Geometry check sheet. Reference: the model listing, model coordinates, mm. A direction names the side the tool comes from. Give positions to 0.01 mm unless a question says otherwise; leave off trailing zeros. Write each loop counter-clockwise with the first axis right and the second up, starting at its lowest first coordinate (ties: lowest second). Pieces come first, ordered by that corner, then holes. Notation, with made-up numbers: (-4.5, -15.5) -> (15.5, -15.5) arc R15 cw to (15.5, -5.5) -> close; hole circle Ø8 at (59.25, -34.75). An arc over 180 degrees is marked (long way). Write item = value, one per line. Start each with the question number.
1. Cross-section at C-C, the plane z = 2.75. Record the cut outline in (x, y).
2. Mould release check, pull along Z, two halves, no side actions. Record for faces 6 (the flat face through (25, -3, 7)), 7 (the flat face through (7, -14, 14)), 8 (the flat face through (21, -6, 7)): pulls with the +Z half, pulls with the -Z half, needs draft (parallel to the pull), parting line crosses it, or undercut.
3. Depth check by flat-ended pin: P1, Ø2, axis at x = 18.5, z = 9.5, coming from the -Y side; P2, Ø2, axis at y = -17.5, z = 6, coming from the +X side; P3, Ø5.5, axis at y = -17.78, z = 7, coming from the -X side; P4, Ø6, axis at x = 13.5, y = -32.5, coming from the +Z side. Enter the tip coordinate at first touch or a pass-through.
4. Cross-section at A-A, the plane z = 7. Record the cut outline in (x, y), plus the area to 3 significant figures.
5. Cross-section at B-B, the plane y = -1. Record the cut outline in (x, z).
6. Thickness scan on line 1 along Y through (x, z) = (2.4, 7); line 2 along Z through (x, y) = (19.5, -16.5); line 3 along X through (y, z) = (-38, 4.25). Record the ranges inside material, lowest first.
7. Set-up check for faces 1 (the flat face through (-9.5, 5, 7)), 2 (the cylindrical face through (8.281, -8.406, 7.074)), 3 (the flat face through (-2, 3, 7)), 4 (the flat face through (16.405, -23.681, 0.838)), 5 (the flat face through (0, -25, 7)): record each of +Z, -Z, +X, -X, +Y, -Y from which the full face is reachable in a straight line by a thin tool's end or side.
8. Cross-section at D-D, the plane x = -11.5. Record the cut outline in (y, z).
```python
from build123d import *

# Parameters (mm, degrees)
BOSS_EXTRUDE1_DEPTH = 14
SKETCH2_R           = 1.7
CUT_EXTRUDE1_DEPTH  = 10
SKETCH3_R           = 1.7
CUT_EXTRUDE2_DEPTH  = 10
SKETCH14_W          = 14
SKETCH14_H          = 6
BOSS_EXTRUDE3_DEPTH = 14
FILLET8_R           = 2
SKETCH17_W          = 1.5
SKETCH17_H          = 1.7
SKETCH18_W          = 19
SKETCH18_H          = 1.7
SKETCH20_W          = 19
SKETCH20_H          = 1.7
SKETCH19_W          = 1.5
SKETCH19_H          = 1.7
FILLET9_R           = 8
SKETCH21_W          = 7.5
SKETCH21_H          = 7
BOSS_EXTRUDE4_DEPTH = 14
FILLET10_R          = 4
FILLET11_R          = 2
FILLET12_R          = 2


with BuildPart() as part:
    # Sketch1 → Boss-Extrude1 (new body)
    with BuildSketch(Plane.XY):
        Polygon((0, 0), (25, 0), (25, -6), (6, -6), (6, -42), (0, -42), (0, -5.547169811), align=None)
    extrude(amount=BOSS_EXTRUDE1_DEPTH)

    # Sketch2 → Cut-Extrude1 (cut)
    with BuildSketch(Plane(origin=(6, 0, 0), x_dir=(0, 0, -1), z_dir=(1, 0, 0))):
        with Locations((-7, -17.78)):
            Circle(SKETCH2_R)
        with Locations((-7, -34.058)):
            Circle(SKETCH2_R)
    extrude(amount=-CUT_EXTRUDE1_DEPTH, mode=Mode.SUBTRACT)

    # Sketch3 → Cut-Extrude2 (cut)
    with BuildSketch(Plane.XZ.offset(6)):
        with Locations((18.3, 7)):
            Circle(SKETCH3_R)
    extrude(amount=-CUT_EXTRUDE2_DEPTH, mode=Mode.SUBTRACT)

    # Sketch14 → Boss-Extrude3 (add)
    with BuildSketch(Plane(origin=(0, 0, 0), x_dir=(-1, 0, 0), z_dir=(0, 0, -1))):
        with Locations((7, -3)):
            Rectangle(SKETCH14_W, SKETCH14_H)
    extrude(amount=-BOSS_EXTRUDE3_DEPTH)

    # Fillet8
    fillet8_edges = [part.edges().sort_by_distance(p)[0] for p in [
        (0, -6, 7),
    ]]
    fillet(fillet8_edges, radius=FILLET8_R)

    # Sketch17 → Loft2 section 0
    with BuildSketch(Plane.XZ.offset(42)):
        with Locations((6.75, 13.15)):
            Rectangle(SKETCH17_W, SKETCH17_H)
    # Sketch18 → Loft2 section 1
    with BuildSketch(Plane.XZ.offset(6)):
        with Locations((15.5, 13.15)):
            Rectangle(SKETCH18_W, SKETCH18_H)
    loft()

    # Sketch20 → Loft3 section 0
    with BuildSketch(Plane.XZ.offset(6)):
        with Locations((15.5, 0.85)):
            Rectangle(SKETCH20_W, SKETCH20_H)
    # Sketch19 → Loft3 section 1
    with BuildSketch(Plane.XZ.offset(42)):
        with Locations((6.75, 0.85)):
            Rectangle(SKETCH19_W, SKETCH19_H)
    loft()

    # Fillet9
    fillet9_edges = [part.edges().sort_by_distance(p)[0] for p in [
        (6, -6, 7),
    ]]
    fillet(fillet9_edges, radius=FILLET9_R)

    # Sketch21 → Boss-Extrude4 (add)
    with BuildSketch(Plane(origin=(0, 0, 0), x_dir=(-1, 0, 0), z_dir=(0, 0, -1))):
        with Locations((5.75, 3.5)):
            Rectangle(SKETCH21_W, SKETCH21_H)
    extrude(amount=-BOSS_EXTRUDE4_DEPTH)

    # Fillet10
    fillet10_edges = [part.edges().sort_by_distance(p)[0] for p in [
        (-9.5, 0, 7),
    ]]
    fillet(fillet10_edges, radius=FILLET10_R)

    # Fillet11
    fillet11_edges = [part.edges().sort_by_distance(p)[0] for p in [
        (7.5, -42, 0.85),
    ]]
    fillet(fillet11_edges, radius=FILLET11_R)

    # Fillet12
    fillet12_edges = [part.edges().sort_by_distance(p)[0] for p in [
        (7.5, -42, 13.15),
    ]]
    fillet(fillet12_edges, radius=FILLET12_R)


solid = part.part
```
Answers:
q1.outline = (-14, -6) -> (-2, -6) arc R2 cw to (0, -8) -> (0, -42) -> (6, -42) -> (6, -14) arc R8 cw to (14, -6) -> (25, -6) -> (25, 0) -> (-2, 0) -> (-2, 7) -> (-9.5, 7) -> (-9.5, 4) arc R4 cw to (-13.5, 0) -> (-14, 0) -> close
q2.face_6 = needs draft
q2.face_7 = pulls with the +Z half
q2.face_8 = undercut
q3.P1 = -6
q3.P2 = 6
q3.P3 = 0
q3.P4 = 14
q4.outline = (-14, -6) -> (-2, -6) arc R2 cw to (0, -8) -> (0, -16.08) -> (6, -16.08) -> (6, -14) arc R8 cw to (14, -6) -> (16.6, -6) -> (16.6, 0) -> (-2, 0) -> (-2, 7) -> (-9.5, 7) -> (-9.5, 4) arc R4 cw to (-13.5, 0) -> (-14, 0) -> close; (0, -42) -> (6, -42) -> (6, -35.76) -> (0, -35.76) -> close; (0, -32.36) -> (6, -32.36) -> (6, -19.48) -> (0, -19.48) -> close; (20, -6) -> (25, -6) -> (25, 0) -> (20, 0) -> close
q4.area = 459 mm^2
q5.outline = (-14, 0) -> (25, 0) -> (25, 14) -> (-14, 14) -> close; hole circle Ø3.4 at (18.3, 7)
q6.line_1 = -42 to -35.76, -32.36 to -19.48, -16.08 to 0
q6.line_2 = 0 to 1.7, 12.3 to 14
q6.line_3 = 0 to 6
q7.face_1 = +Z, -Z, -X, +Y
q7.face_2 = +X, -Y
q7.face_3 = +Z, -Z, +X, +Y
q7.face_4 = +Z, -Z, +X, -Y
q7.face_5 = +Z, -Z, -X, -Y
q8.outline = (-6, 0) -> (0.54, 0) -> (0.54, 14) -> (-6, 14) -> close
